Check sheet for the modelled part. Datum: model origin and axes. Units: mm. Face numbers are marked on the shaded views. A direction names the side the tool comes from. Coordinates: 2 decimals unless noted, no trailing zeros. Write each loop counter-clockwise with the first axis right and the second up, starting at its lowest first coordinate (ties: lowest second). Pieces come first, ordered by that corner, then holes. Notation, with made-up numbers: (43, 40.25) -> (97, 40.25) arc R25 ccw to (97, 69.25) -> close; hole circle Ø7 at (25, 57.25). An arc over 180 degrees is marked (long way). Put each result on its own line as item: value.
```python
from build123d import *

# Parameters (mm, degrees)
SKETCH_1_W          = 26
SKETCH_1_H          = 20
EXTRUDE_1_DEPTH     = 25
CUT_EXTRUDE_1_DEPTH = 16
FILLET_1_R          = 2
SKETCH_3_R          = 1.25
CUT_EXTRUDE_2_DEPTH = 23.912878475
SKETCH_4_R          = 1.65
CUT_EXTRUDE_3_DEPTH = 35.554305086
SKETCH_5_W          = 20
SKETCH_5_H          = 5
CUT_EXTRUDE_4_DEPTH = 38.429934544
SKETCH_6_W          = 26
SKETCH_6_H          = 10
CUT_EXTRUDE_5_DEPTH = 35.554305086
SKETCH_7_W          = 2
SKETCH_7_H          = 1
EXTRUDE_2_DEPTH     = 10


with BuildPart() as part:
    # 草图1 → 凸台-拉伸1 (new body)
    with BuildSketch(Plane(origin=(0, 0, 0), x_dir=(1, 0, 0), z_dir=(0, 1, 0))):
        Rectangle(SKETCH_1_W, SKETCH_1_H)
    extrude(amount=EXTRUDE_1_DEPTH)

    # 草图2 → 切除-拉伸1 (cut)
    with BuildSketch(Plane.XZ):
        with BuildLine():
            Line((5, 2.06571985), (5, -10))
            Line((5, -10), (7, -10))
            Line((7, -10), (7, 2.06571985))
            ThreePointArc((7, 2.06571985), (6, 8.1), (5, 2.06571985))
        make_face()
    extrude(amount=-CUT_EXTRUDE_1_DEPTH, mode=Mode.SUBTRACT)

    # 圆角1
    fillet_1_edges = [part.edges().sort_by_distance(p)[0] for p in [
        (5, 8, 2.06571985),
        (7, 8, 2.06571985),
    ]]
    fillet(fillet_1_edges, radius=FILLET_1_R)

    # 草图3 → 切除-拉伸2 (cut, through all)
    with BuildSketch(Plane.XZ.offset(-16)):
        with Locations(Location((6, 5, 0), (0, 0, 270))):
            Circle(SKETCH_3_R)
    extrude(amount=-CUT_EXTRUDE_2_DEPTH, mode=Mode.SUBTRACT)

    # 草图4 → 切除-拉伸3 (cut, through all)
    with BuildSketch(Plane(origin=(0, 0, -10), x_dir=(-1, 0, 0), z_dir=(0, 0, -1))):
        with Locations((8, 10.5)):
            Circle(SKETCH_4_R)
        with Locations((0, 10.5)):
            Circle(SKETCH_4_R)
    extrude(amount=-CUT_EXTRUDE_3_DEPTH, mode=Mode.SUBTRACT)

    # 草图5 → 切除-拉伸4 (cut, through all)
    with BuildSketch(Plane(origin=(13, 0, 0), x_dir=(0, 0, -1), z_dir=(1, 0, 0))):
        with Locations((0, 2.5)):
            Rectangle(SKETCH_5_W, SKETCH_5_H)
    extrude(amount=-CUT_EXTRUDE_4_DEPTH, mode=Mode.SUBTRACT)

    # 草图6 → 切除-拉伸5 (cut, through all)
    with BuildSketch(Plane(origin=(0, 0, -10), x_dir=(-1, 0, 0), z_dir=(0, 0, -1))):
        with Locations((0, 20)):
            Rectangle(SKETCH_6_W, SKETCH_6_H)
    extrude(amount=-CUT_EXTRUDE_5_DEPTH, mode=Mode.SUBTRACT)

    # 草图7 → 凸台-拉伸2 (add)
    with BuildSketch(Plane(origin=(0, 15, 0), x_dir=(1, 0, 0), z_dir=(0, 1, 0))):
        with Locations((6, 9.5)):
            Rectangle(SKETCH_7_W, SKETCH_7_H)
    extrude(amount=-EXTRUDE_2_DEPTH)


solid = part.part
```
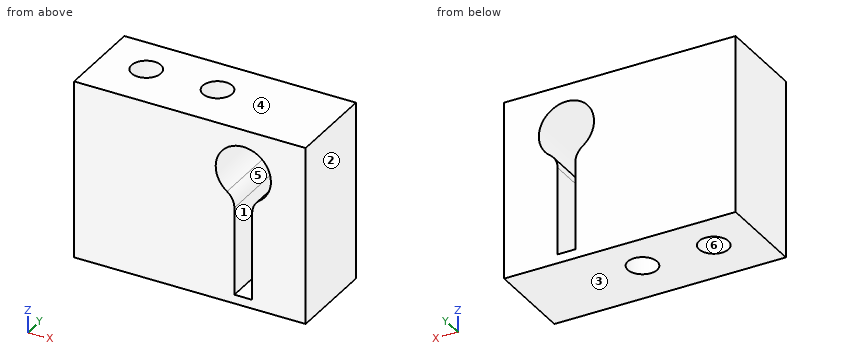
Q1. Cross-section at B-B (y = 10.5). Record the cut outline in (x, z), plus the area to 3 significant figures.
Recorded:
outline: (-13, -10) -> (-9.65, -10) -> (-9.65, 10) -> (-13, 10) -> close; (-6.35, -10) -> (-1.65, -10) -> (-1.65, 10) -> (-6.35, 10) -> close; (1.65, -10) -> (13, -10) -> (13, 10) -> (1.65, 10) -> close; hole (4.18, 2.49) arc R2 cw to (5, 0.88) -> (5, -9) -> (7, -9) -> (7, 0.88) arc R2 cw to (7.82, 2.49) arc R3.1 ccw (long way) to start
area: 335 mm2
Q2. Tool access check on the marked faces 5 and 6. Record the directions out of +Z, -Z, +X, -X, +Y, -Y that give a thin tool (end or side, any length) a straight path to the whole face; none if there is none.
Recorded:
face 5: +Y, -Y
face 6: +Z, -Z
Q3. Cross-section at D-D (z = -1.5). Record the cut outline in (x, y).
Recorded:
outline: (-13, 5) -> (5, 5) -> (5, 15) -> (-13, 15) -> close; (7, 5) -> (13, 5) -> (13, 15) -> (7, 15) -> close; hole circle Ø3.3 at (-8, 10.5); hole circle Ø3.3 at (0, 10.5)
Q4. Material ranges on line 1 along Y through (x, z) = (0, 3.25); line 2 along X through (y, z) = (8.5, 5); line 3 along X through (y, z) = (9.25, 9), recorded low to high.
Recorded:
line 1: y = 5 to 8.85, 12.15 to 15
line 2: x = -13 to 2.9, 9.1 to 13
line 3: x = -13 to -9.08, -6.92 to -1.08, 1.08 to 13
Q5. Cross-section at C-C (x = 0). Record the cut outline in (y, z).
Recorded:
outline: (5, -10) -> (8.85, -10) -> (8.85, 10) -> (5, 10) -> close; (12.15, -10) -> (15, -10) -> (15, 10) -> (12.15, 10) -> close
Q6. Depth check by flat-ended pin: P1, Ø2.5, axis at x = -8, y = 10.5, coming from the -Z side. Enter the tip coordinate at first touch or a pass-through.
Recorded:
P1: passes through
Q7. Mould release check, pull along Z, two halves, no side actions. Record for the marked faces 1, 2, 3 and 4: released by +Z, released by -Z, zero draft, split by the parting line, or undercut.
Recorded:
face 1: undercut
face 2: zero draft
face 3: released by -Z
face 4: released by +Z
Q8. Cross-section at A-A (z = 5). Record the cut outline in (x, y).
Recorded:
outline: (-13, 5) -> (2.9, 5) -> (2.9, 15) -> (-13, 15) -> close; (9.1, 5) -> (13, 5) -> (13, 15) -> (9.1, 15) -> close; hole circle Ø3.3 at (-8, 10.5); hole circle Ø3.3 at (0, 10.5)
